Could you check a few things on this model? Use its own coordinates, in mm. Face numbers are marked on the shaded views. A direction names the side the tool comes from. Give positions to 0.01 mm unless a question says otherwise; leave off trailing zeros. Loops run counter-clockwise (first coordinate to the right, second up) from the corner with the lowest first, then second, coordinate; pieces in that order, holes last. Notation, with made-up numbers: (13.25, 18) - (17.25, 18) arc R21 ccw to (17.25, 30) - close; hole circle Ø6 at (16, 75). An arc over 180 degrees is marked (long way). One line per item, written item: value. Start each with the question number.
Q1. I want a section at B-B (x = 29.5). Please give me the cut outline in (y, z).
Q2. I want a section at A-A (z = -29.5). Please give me the cut outline in (x, y), then the cut area to 3 significant figures.
Q3. If I drill on line 1 (Z direction, x = 0, y = 9); line 2 (X direction, y = 9, z = 112); line 3 (Y direction, x = 25, z = 80.5), over which ranges is the centre line in solid material (lowest first)? Write a range as from..to.
Q4. I want a section at C-C (y = 37). Please give me the cut outline in (x, z).
Q5. I'm going to push flat-ended pins straight in: P1, Ø10, axis at x = -49.5, z = -16, coming from the +Y side; P2, Ø5, axis at y = 22, z = -110.5, coming from the +X side. Where does each tip first touch, or does it pass through?
Q6. For the marked faces 1 and 2, which set-ups out of +Z, -Z, +X, -X, +Y, -Y let a thin tool reach every point of the face, with its end or its side?
```python
from build123d import *

# Parameters (mm, degrees)
SKETCH1_W             = 150
SKETCH1_H             = 300
BOSS_EXTRUDE1_DEPTH   = 16
SKETCH2_W             = 16
SKETCH2_H             = 300
BOSS_EXTRUDE2_DEPTH   = 25
FILLET1_R             = 10
F_8_36_TAPPED_HOLE1_D = 3.4544


with BuildPart() as part:
    # Sketch1 → Boss-Extrude1 (new body)
    with BuildSketch(Plane(origin=(0, 0, 0), x_dir=(1, 0, 0), z_dir=(0, 1, 0))):
        Rectangle(SKETCH1_W, SKETCH1_H)
    extrude(amount=BOSS_EXTRUDE1_DEPTH)

    # Sketch2 → Boss-Extrude2 (add)
    with BuildSketch(Plane(origin=(0, 16, 0), x_dir=(1, 0, 0), z_dir=(0, 1, 0))):
        with Locations((-67, 0)):
            Rectangle(SKETCH2_W, SKETCH2_H)
    extrude(amount=BOSS_EXTRUDE2_DEPTH)

    # Fillet1
    fillet1_edges = [part.edges().sort_by_distance(p)[0] for p in [
        (-59, 41, 0),
    ]]
    fillet(fillet1_edges, radius=FILLET1_R)

    # #8-36 Tapped Hole1 (through all)
    with Locations(Plane(origin=(0, 0, 0), x_dir=(-1, 0, 0), z_dir=(0, -1, 0))):
        with Locations((0, 112), (0, 88)):
            f_8_36_tapped_hole1 = Hole(F_8_36_TAPPED_HOLE1_D / 2)

    # Mirror1: #8-36 Tapped Hole1 across plane
    add(f_8_36_tapped_hole1.mirror(Plane.XY), mode=Mode.SUBTRACT)


solid = part.part
```
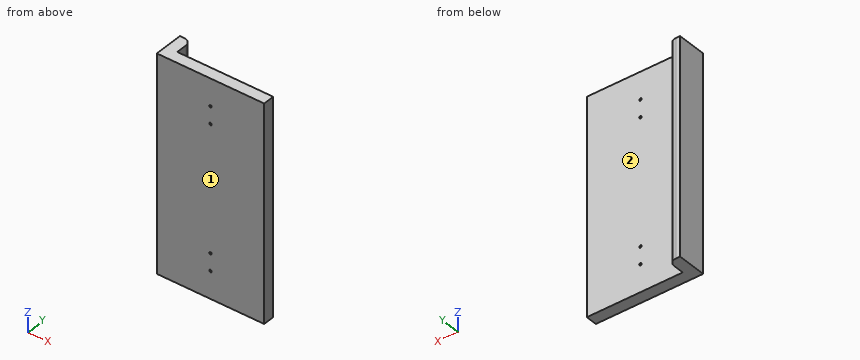
Worked answers:
1. outline: (0, -150) - (16, -150) - (16, 150) - (0, 150) - close
2. outline: (-75, 0) - (75, 0) - (75, 16) - (-59, 16) - (-59, 31) arc R10 ccw to (-69, 41) - (-75, 41) - close
2. area: 2,780 mm²
3. line 1: z = -150..-113.73, -110.27..-89.73, -86.27..86.27, 89.73..110.27, 113.73..150
3. line 2: x = -75..-1.73, 1.73..75
3. line 3: y = 0..16
4. outline: (-75, -150) - (-61, -150) - (-61, 150) - (-75, 150) - close
5. P1: stops at y = 16
5. P2: stops at x = -59
6. face 1: +Z, -Z, +X, -X, -Y
6. face 2: +Z, -Z, +X, +Y
